Input: part model. Units: mm. Frame: model coordinates. Round coordinates to 2 decimals unless told otherwise and drop trailing zeros. Loops run counter-clockwise (first coordinate to the right, second up) from the corner with the lowest first, then second, coordinate; pieces in that order, holes last.
(1) Draft query along Z for faces 1 (the face through (2, 0, 7)), 2 (the face through (-4.31, 1.972, 7.327)), 3 (the face through (0.19, 0.02, -8.72)), 4 (the face through (3.472, 1.98, 5.446)). Return one class per face: released by +Z, released by -Z, zero draft, split by the parting line, or undercut.
(2) Cut plane A-A, the plane y = 2.5. Output: boundary loops of the cut face in (x, z) (1 decimal), and give its area (3 significant figures).
(3) First-contact query: pin 1 Ø2 at (x, y) = (3, 2.5) entering from -Z; pin 2 Ø2 at (x, y) = (4, 3.5) entering from +Z; pin 3 Ø1.5 at (x, y) = (-1.5, 3.5) entering from -Z. Flat tips, straight axial feed; report the tip coordinate or a pass-through.
(4) Line query: line 1 (X direction, y = 2.3, z = 0.25); line 2 (Z direction, x = -5.25, y = 2.3); line 3 (Z direction, x = -5.5, y = 3.4). Output: solid intervals per line, ascending.
Autodesk Inventor part; units mm, degrees
ref_plane "ANBAU_XY" through (0, 0, 0) normal (0, 1, 0) x (1, 0, 0)
ref_plane "ANBAU_YZ" through (0, 0, 0) normal (1, 0, 0) x (0, 0, -1)
ref_plane "ANBAU_ZX" through (0, 0, 0) normal (0, 0, -1) x (0, 1, 0)
sketch "Skizze_1" plane through (0, 0, 0) normal (0, 0, 1) x (1, 0, 0)
  line L0 (0, 0) -> (0, 4)
  line L1 (0, 4) -> (8.5, 4)
  line L2 (8.5, 4) -> (12.75, 3.6282)
  line L3 (12.75, 3.6282) -> (12.75, 0.3718)
  line L4 (12.75, 0.3718) -> (8.5, 0)
  line L5 (8.5, 0) -> (0, 0)
  line L6 (0, 0) -> (0, 4)
revolve "Revolution1" add sketch "Skizze_1" angle 360 about axis through (0, 0, 0) along (0, -1, 0)
sketch "Skizze_2" plane through (0, 4, 0) normal (0, 1, 0) x (1, 0, 0)
  line L0 (-17, 17) -> (-17, -17)
  line L1 (-17, -17) -> (17, -17)
  line L2 (17, -17) -> (17, 17)
  line L3 (17, 17) -> (-17, 17)
  line L4 (-8.5, -4.9075) -> (0, -9.815)
  line L5 (0, -9.815) -> (8.5, -4.9075)
  line L6 (8.5, -4.9075) -> (8.5, 4.9075)
  line L7 (8.5, 4.9075) -> (0, 9.815)
  line L8 (0, 9.815) -> (-8.5, 4.9075)
  line L9 (-8.5, 4.9075) -> (-8.5, -4.9075)
extrude "Extrusion1" cut sketch "Skizze_2" along normal mid plane 8
sketch "Sketch_1" plane through (0, 0, 0) normal (0, 0, 1) x (1, 0, 0)
  line L0 (0, 0) -> (0, 4)
  line L1 (0, 4) -> (7, 4)
  line L2 (7, 4) -> (6.4585, 3.4585)
  line L3 (6.4585, 3.4585) -> (6.4585, 0.5415)
  line L4 (6.4585, 0.5415) -> (7, 0)
  line L5 (7, 0) -> (0, 0)
  line L6 (0, 0) -> (0, 4)
revolve "Revolution2" cut sketch "Sketch_1" angle 360 about axis through (0, 0, 0) along (0, -1, 0)
thread "Thread1"
ref_plane "ANBAU_XY" through (0, 0, 0) normal (0, 1, 0) x (1, 0, 0)
ref_plane "ANBAU_YZ" through (0, 0, 0) normal (1, 0, 0) x (0, 0, -1)
ref_plane "ANBAU_ZX" through (0, 0, 0) normal (0, 0, -1) x (0, 1, 0)
properties part number "130519 ESHM-M14x1"
Reported:
1. face 1: zero draft
1. face 2: released by +Z
1. face 3: released by -Z
1. face 4: undercut
2. outline: (-8.5, -4.9) - (0, -9.8) - (8.5, -4.9) - (8.5, 4.9) - (0, 9.8) - (-8.5, 4.9) - close; hole circle Ø12.9 at (0, 0)
2. area: 119 mm2
3. pin 1: stops at z = -8.66
3. pin 2: stops at z = 8.08
3. pin 3: stops at z = -9.38
4. line 1: x = -8.5 to -6.45, 6.45 to 8.5
4. line 2: z = -6.78 to -3.76, 3.76 to 6.78
4. line 3: z = -6.64 to -3.39, 3.39 to 6.64
